Geometry: see drawing. Coordinates: mm, zero at the bounding-box minimum. A direction names the side the tool comes from. Round coordinates to 2 decimals unless told otherwise and drop trailing zeros. Order: outer loops, then holes, each group sorted by start corner. A loop starts at its lowest first (then second) coordinate and runs counter-clockwise, first axis right, second up. Notation, with made-up numbers: (76.25, -8.5) -> (81.25, -8.5) arc R23 ccw to (81.25, 11.5) -> close; hole circle Ø10 at (53.25, 57.5). An arc over 180 degrees is marked (long way). One line per item, written item: value. Start each with the question number.
1) Pin query (flat end, axial travel): P1, Ø5, axis at x = 23.5, y = 17, coming from the -Z side (3 decimals); P2, Ø8, axis at x = 21.5, y = 25, coming from the +Z side (3 decimals); P3, Ø4, axis at x = 25, z = 78.5, coming from the +Y side (3 decimals). Return the tip coordinate at first contact, or that it passes through.
2) Section A-A (y = 6.5). Return the cut outline in (x, z), and give its area (3 significant figures).
3) Section C-C (x = 3). Return the cut outline in (y, z) (1 decimal), and give its area (3 significant figures).
4) Section B-B (x = 16). Return the cut outline in (y, z) (3 decimals), and give its area (3 significant figures).
5) Reachability of the marked faces 1, 2 and 3 from +Z, -Z, +X, -X, +Y, -Y: full face, straight path, thin tool, end or side. Return the list, or none.
6) Ray query, L1, parallel to Z at x = 32, y = 27 (3 decimals); L2, parallel to Y at x = 3, z = 77 (3 decimals). Return the intervals inside material, ascending.
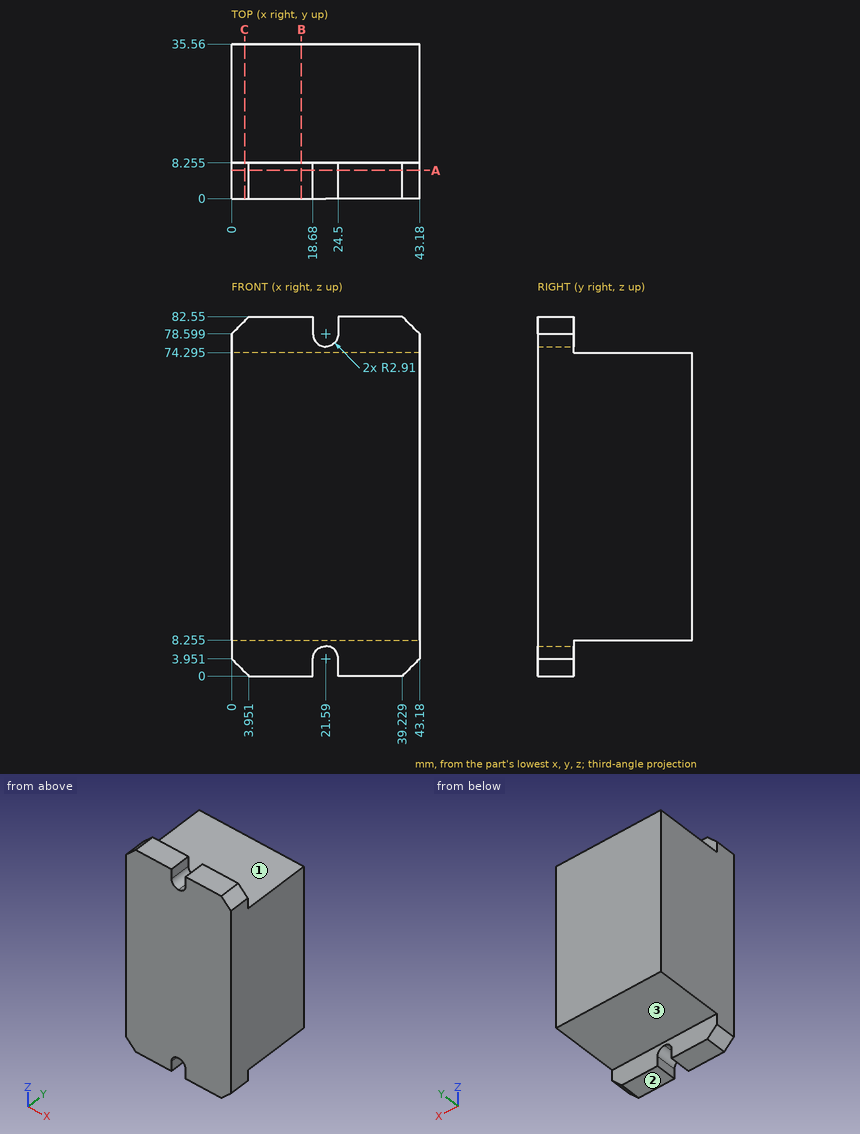
Findings:
1. P1: z = 8.255
1. P2: z = 74.295
1. P3: y = 8.255
2. outline: (0, 3.95) -> (3.95, 0) -> (18.68, 0) -> (18.68, 3.95) arc R2.91 cw to (24.5, 3.95) -> (24.5, 0) -> (39.23, 0) -> (43.18, 3.95) -> (43.18, 78.6) -> (39.23, 82.55) -> (24.5, 82.55) -> (24.5, 78.6) arc R2.91 cw to (18.68, 78.6) -> (18.68, 82.55) -> (3.95, 82.55) -> (0, 78.6) -> close
2. area: 3,460 mm2
3. outline: (0, 1) -> (8.3, 1) -> (8.3, 8.3) -> (35.6, 8.3) -> (35.6, 74.3) -> (8.3, 74.3) -> (8.3, 81.6) -> (0, 81.6) -> close
3. area: 2,470 mm2
4. outline: (0, 0) -> (8.255, 0) -> (8.255, 8.255) -> (35.56, 8.255) -> (35.56, 74.295) -> (8.255, 74.295) -> (8.255, 82.55) -> (0, 82.55) -> close
4. area: 2,480 mm2
5. face 1: +Z, +X, -X, +Y
5. face 2: -Z, +X, -X, +Y, -Y
5. face 3: -Z, +X, -X, +Y
6. L1: 8.255 to 74.295
6. L2: 0 to 8.255
